from build123d import *

# Parameters (mm, degrees)
F1_DEPTH = 10
F2_R     = 1
F2_W     = 0.686881559
F2_H     = 10
F3_DEPTH = 1


with BuildPart() as f1:
    # F0 (on Top) → F1 (new body)
    with BuildSketch(Plane.XY):
        with BuildLine():
            Line((1.5, 2), (4.0311288741, 2))
            ThreePointArc((4.0311288741, 2), (-4.5, 0), (4.0311288741, -2))
            Line((4.0311288741, -2), (1.5, -2))
            ThreePointArc((1.5, -2), (-2.5, 0), (1.5, 2))
        make_face()
    extrude(amount=F1_DEPTH)

    # F2 (on Front) → F3 (join, symmetric)
    with BuildSketch(Plane.XZ):
        with BuildLine():
            Line((-4.5, 10), (-7.732233047, 6.767766953))
            ThreePointArc((-7.732233047, 6.767766953), (-8.4644660941, 5), (-7.732233047, 3.232233047))
            Line((-7.732233047, 3.232233047), (-4.5, 0))
            Line((-4.5, 0), (-4.5, 10))
        make_face()
        with Locations((-5.9644660941, 5)):
            Circle(F2_R, mode=Mode.SUBTRACT)
        with Locations((-4.1565592205, 5)):
            Rectangle(F2_W, F2_H)
    extrude(amount=F3_DEPTH, both=True)


solid = f1.part
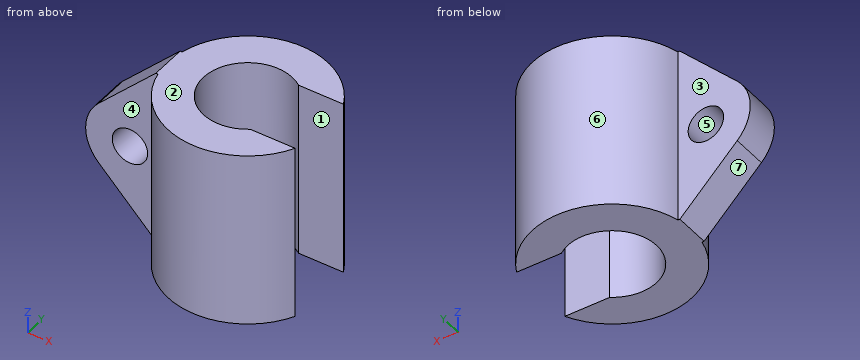
Input: part model. Units: mm. Frame: model coordinates. Face numbers are marked on the shaded views. A direction names the side the tool comes from. Give positions to 0.01 mm unless a question says otherwise; leave off trailing zeros. Order: outer loops, then holes, each group sorted by start corner. A loop starts at its lowest first (then second) coordinate and runs counter-clockwise, first axis right, second up.
Q1. Draft query along Z for the marked faces 5, 6 and 7. Return one class per face: +Z half, -Z half, draft (parallel to the pull), parting line (faces both ways), or undercut.
Checked values:
face 5: undercut
face 6: draft
face 7: -Z half
Q2. Ray query, probe 1 along Y at (x, z) = (0, 6.75); probe 2 along Y at (x, z) = (2, 6.25); probe 3 along X at (y, z) = (0.5, 4.25). Return the intervals inside material, ascending.
Checked values:
probe 1: y = -4.5 to -2.5, 2.5 to 4.5
probe 2: y = -4.03 to -2, 2 to 4.03
probe 3: x = -8.35 to -6.63, -5.3 to -2.45
Q3. Section D-D on z = 2.5. Output: boundary loops of the cut face in (x, y), and give its area (3 significant figures).
Checked values:
outline: (-7, -1) - (-4.39, -1) arc R4.5 ccw to (4.03, -2) - (1.5, -2) arc R2.5 cw (long way) to (1.5, 2) - (4.03, 2) arc R4.5 ccw to (-4.39, 1) - (-7, 1) - close
area: 40.5 mm2
Q4. Section B-B on y = 0. Output: boundary loops of the cut face in (x, z).
Checked values:
outline: (-7.73, 3.23) - (-4.5, 0) - (-2.5, 0) - (-2.5, 10) - (-4.5, 10) - (-7.73, 6.77) arc R2.5 ccw to start; hole circle Ø2 at (-5.96, 5)
Q5. Section C-C on z = 5. Output: boundary loops of the cut face in (x, y).
Checked values:
outline: (-8.46, -1) - (-6.96, -1) - (-6.96, 1) - (-8.46, 1) - close; (-4.96, -1) - (-4.39, -1) arc R4.5 ccw to (4.03, -2) - (1.5, -2) arc R2.5 cw (long way) to (1.5, 2) - (4.03, 2) arc R4.5 ccw to (-4.39, 1) - (-4.96, 1) - close
Q6. Section A-A on x = 0. Output: boundary loops of the cut face in (y, z), and give its area (3 significant figures).
Checked values:
outline: (-4.5, 0) - (-2.5, 0) - (-2.5, 10) - (-4.5, 10) - close; (2.5, 0) - (4.5, 0) - (4.5, 10) - (2.5, 10) - close
area: 40.0 mm2
Q7. Set-up query: the marked faces 1, 2, 3 and 4. Return all of +Z, -Z, +X, -X, +Y, -Y with unobstructed straight access to the full face (end or side cutting, diameter ignored); none if empty.
Checked values:
face 1: +Z, -Z, +X
face 2: +Z, +X, -X, +Y, -Y
face 3: +Z, -Z, -X, +Y
face 4: +Z, -Z, -X, -Y
Q8. Contact query for flat-ended pins moving along their axis: pin 1 Ø1.6 at (x, z) = (-5.96, 5) entering from -Y; pin 2 Ø0.8 at (x, z) = (2.5, 6.5) entering from -Y; pin 3 Ø2 at (x, z) = (-7.5, 2.5) entering from +Y; pin 4 Ø2 at (x, z) = (-7, 5.5) entering from -Y. Output: stop coordinate, or through.
Checked values:
pin 1: passes through
pin 2: stops at y = -3.98
pin 3: stops at y = 1
pin 4: stops at y = -1
